Autodesk Inventor part; units mm, degrees
ref_plane "YZ Plane" through (0, 0, 0) normal (1, 0, 0) x (0, 1, 0)
ref_plane "XZ Plane" through (0, 0, 0) normal (0, 1, 0) x (-1, 0, 0)
ref_plane "XY Plane" through (0, 0, 0) normal (0, 0, 1) x (1, 0, 0)
sketch "Sketch1" plane through (0, 0, 0) normal (0, 0, 1) x (1, 0, 0)
  circle A0 centre (0, 0) radius 5.7
  dimension "d0" = 11.4
extrude "Extrusion1" add sketch "Sketch1" along normal blind 30
chamfer "Chamfer1" distance 0.8 angle 45 1 edges at (-5.7, 0, 30)
sketch "Sketch2" plane through (0, 0, 0) normal (0, 0, 1) x (1, 0, 0)
  circle A0 centre (0, 0) radius 2.9
  dimension "d6" = 5.8
extrude "Extrusion2" cut sketch "Sketch2" along normal up to surface (30 mm away)
properties part number "Insert30mm"
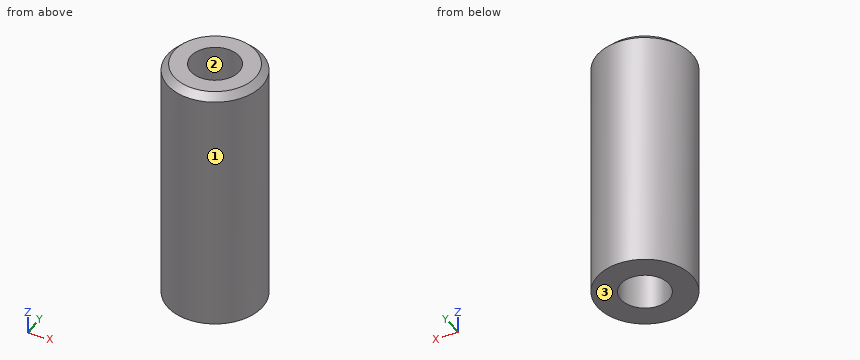
Geometry: final body of the model. Coordinates: model frame, mm. Face numbers are marked on the shaded views. Coordinates: 2 decimals unless noted, no trailing zeros. Order: outer loops, then holes, each group sorted by start corner. A loop starts at its lowest first (then second) coordinate and runs counter-clockwise, first axis right, second up. Notation, with made-up numbers: (74.25, -37) -> (107.25, -37) arc R26 cw to (107.25, -3) -> close; hole circle Ø11 at (-26, 79.25). An arc over 180 degrees is marked (long way). Write each question's results on one line, items separated by ' | '. Start each with the question number.
1) Mould query, pull axis Y, two halves, no side actions, for the marked faces 1, 2 and 3. Classes: released by +Y, released by -Y, zero draft, split by the parting line, or undercut.
2) Material intervals for line 1 along Y through (x, z) = (0, 9.5); line 2 along Y through (x, z) = (-1.25, 5.25); line 3 along X through (y, z) = (-0.75, 25.5), sorted ascending.
3) Cut plane C-C, the plane z = 10.75. Output: boundary loops of the cut face in (x, y), and give its area (3 significant figures).
4) First-contact query: pin 1 (4 mm diameter, centred on x = -3, y = 3.5, fed in from -Z); pin 2 (4 mm diameter, centred on x = -4, z = 25, fed in from -Y); pin 3 (5 mm diameter, centred on x = 3, z = 6, fed in from -Y). Flat tips, straight axial feed; report the tip coordinate or a pass-through.
5) Cut plane A-A, the plane x = 0. Output: boundary loops of the cut face in (y, z), and give its area (3 significant figures).
Checks:
1) face 1: split by the parting line | face 2: undercut | face 3: zero draft
2) line 1: -5.7 to -2.9, 2.9 to 5.7 | line 2: -5.56 to -2.62, 2.62 to 5.56 | line 3: -5.65 to -2.8, 2.8 to 5.65
3) outline: circle Ø11.4 at (0, 0); hole circle Ø5.8 at (0, 0) | area: 75.6 mm^2
4) pin 1: z = 0 | pin 2: y = -5.34 | pin 3: y = -5.68
5) outline: (-5.7, 0) -> (-2.9, 0) -> (-2.9, 30) -> (-4.9, 30) -> (-5.7, 29.2) -> close; (2.9, 0) -> (5.7, 0) -> (5.7, 29.2) -> (4.9, 30) -> (2.9, 30) -> close | area: 167 mm^2
